For this review, take the finished solid that the model builds, in its own axes (mm). Coordinates: 2 decimals unless noted, no trailing zeros. Write each loop counter-clockwise with the first axis right and the second up, starting at its lowest first coordinate (ties: lowest second). Pieces come first, ordered by that corner, then holes.
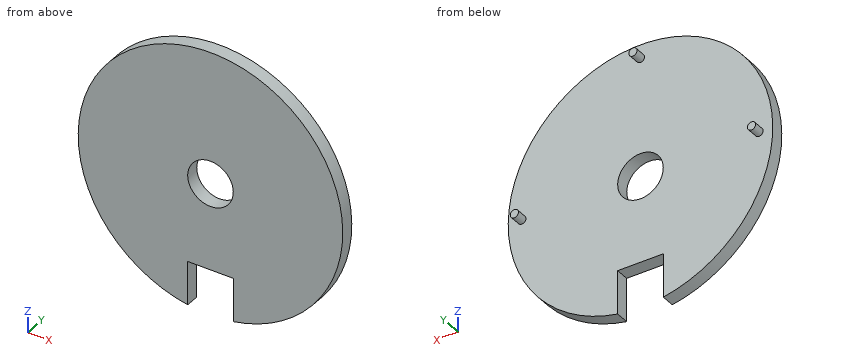
```python
from build123d import *

# Parameters (mm, degrees)
SKETCH1_R           = 29
BOSS_EXTRUDE1_DEPTH = 3
SKETCH6_R           = 0.9
BOSS_EXTRUDE3_DEPTH = 2.5
SKETCH7_R           = 0.9
BOSS_EXTRUDE4_DEPTH = 2.5
SKETCH8_R           = 5
CUT_EXTRUDE2_DEPTH  = 3
CUT_EXTRUDE3_DEPTH  = 10


with BuildPart() as part:
    # Sketch1 → Boss-Extrude1 (new body)
    with BuildSketch(Plane(origin=(0, 0, 0), x_dir=(1, 0, 0), z_dir=(0, 1, 0))):
        with Locations(Location((0, 0, 0), (0, 0, 270))):
            Circle(SKETCH1_R)
    extrude(amount=BOSS_EXTRUDE1_DEPTH)

    # Sketch6 → Boss-Extrude3 (add)
    with BuildSketch(Plane(origin=(0, 3, 0), x_dir=(1, 0, 0), z_dir=(0, 1, 0))):
        with Locations(Location((-26, 0, 0), (0, 0, 270))):
            Circle(SKETCH6_R)
        with Locations(Location((26, 0, 0), (0, 0, 270))):
            Circle(SKETCH6_R)
    extrude(amount=BOSS_EXTRUDE3_DEPTH)

    # Sketch7 → Boss-Extrude4 (add)
    with BuildSketch(Plane(origin=(0, 3, 0), x_dir=(1, 0, 0), z_dir=(0, 1, 0))):
        with Locations(Location((0, -26, 0), (0, 0, 270))):
            Circle(SKETCH7_R)
    extrude(amount=BOSS_EXTRUDE4_DEPTH)

    # Sketch8 → Cut-Extrude2 (cut)
    with BuildSketch(Plane(origin=(0, 3, 0), x_dir=(1, 0, 0), z_dir=(0, 1, 0))):
        with Locations(Location((0, 0, 0), (0, 0, 270))):
            Circle(SKETCH8_R)
    extrude(amount=-CUT_EXTRUDE2_DEPTH, mode=Mode.SUBTRACT)

    # Sketch9 → Cut-Extrude3 (cut)
    with BuildSketch(Plane(origin=(0, 3, 0), x_dir=(1, 0, 0), z_dir=(0, 1, 0))):
        Polygon((0, 29), (5, 29), (5, 19), (-5, 19), (-5, 29), align=None)
    extrude(amount=-CUT_EXTRUDE3_DEPTH, mode=Mode.SUBTRACT)


solid = part.part
```
Q1. Add section B-B (y = 1.6). State the section outline as (x, z) points.
Ans:
outline: (-5, -28.57) - (-5, -19) - (5, -19) - (5, -28.57) arc R29 ccw (long way) to start; hole circle Ø10 at (0, 0)
Q2. Clearance check with flat-ended pins moving along their axes: pin 1 Ø0.9 at (x, y) = (-2.5, 2) entering from -Z; pin 2 Ø6 at (x, z) = (6, -15) entering from -Y; pin 3 Ø1.5 at (y, z) = (2, -23) entering from -X; pin 4 Ø8 at (x, z) = (0, 0) entering from -Y. State where each tip first meets the part, or that it passes through.
Ans:
pin 1: stops at z = -19
pin 2: stops at y = 0
pin 3: stops at x = -18.6
pin 4: passes through
Q3. Add section D-D (z = 26). State the section outline as (x, y) points.
Ans:
outline: (-12.85, 0) - (12.85, 0) - (12.85, 3) - (0.9, 3) - (0.9, 5.5) - (-0.9, 5.5) - (-0.9, 3) - (-12.85, 3) - close
Q4. Add section C-C (x = 3.5). State the section outline as (y, z) points, then the cut area to 3 significant figures.
Ans:
outline: (0, -19) - (3, -19) - (3, -3.57) - (0, -3.57) - close; (0, 3.57) - (3, 3.57) - (3, 28.79) - (0, 28.79) - close
area: 122 mm2
Q5. Add section A-A (z = 0). State the section outline as (x, y) points, then the cut area to 3 significant figures.
Ans:
outline: (-29, 0) - (-5, 0) - (-5, 3) - (-25.1, 3) - (-25.1, 5.5) - (-26.9, 5.5) - (-26.9, 3) - (-29, 3) - close; (5, 0) - (29, 0) - (29, 3) - (26.9, 3) - (26.9, 5.5) - (25.1, 5.5) - (25.1, 3) - (5, 3) - close
area: 153 mm2
Q6. For probe 1 along X at (y, z) = (0.8, 0); probe 2 along Y at (x, z) = (-1, 17); probe 3 along Z at (x, y) = (-10.5, 2.8), list the stretches that pass through material, from the lowest coordinate up.
Ans:
probe 1: x = -29 to -5, 5 to 29
probe 2: y = 0 to 3
probe 3: z = -27.03 to 27.03
